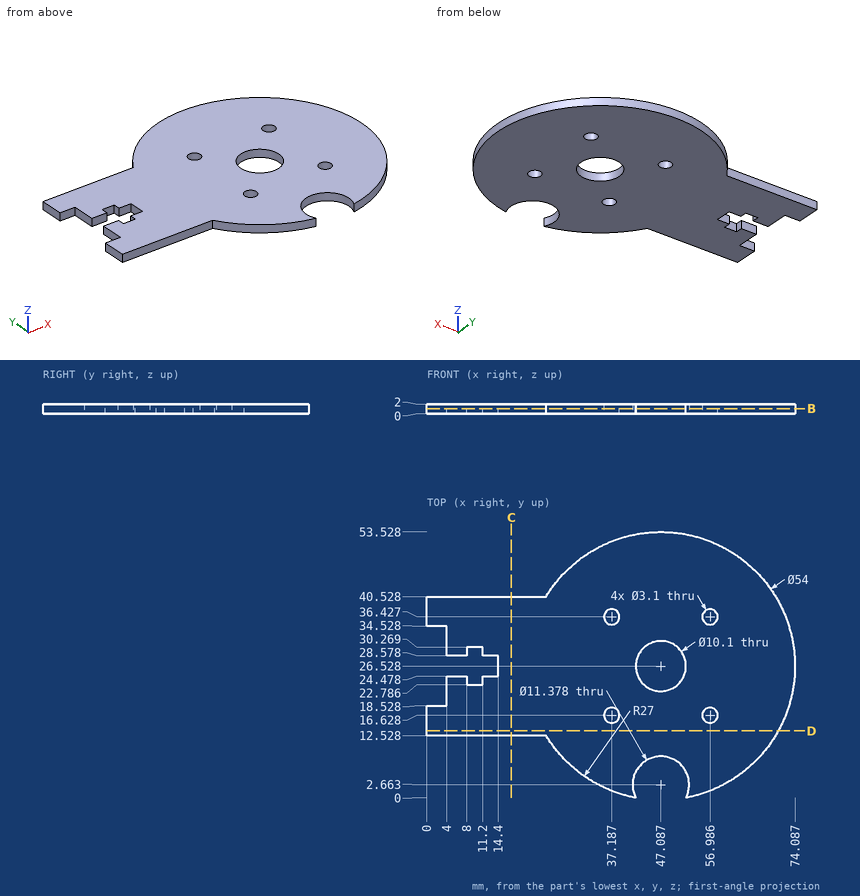
Print and shaded views of the part. All mm, measured from the part's lowest x, y and z. Round coordinates to 2 decimals unless told otherwise and drop trailing zeros. Write each loop counter-clockwise with the first axis right and the second up, starting at its lowest first coordinate (ties: lowest second). Pieces come first, ordered by that corner, then holes. Notation, with made-up numbers: M 84.25,70 L 141.25,70 A16 ccw 141.25,92 Z; hole C 52,87 d2. An arc over 180 degrees is marked long. Use a Markdown table: item, result. Add a question column.
1. Slice it at C-C on x = 17. Give the cut face in (y, z).
2. Drill centre lines: probe 1 along X at (y, z) = (37, 1) (1 decimal); probe 2 along Y at (x, z) = (5.5, 0.7); probe 3 along X at (y, z) = (37.5, 1.25) (1 decimal). Where is each one in solid material? Low to high.
3. Flat gauge pins, fed straight in: P1, Ø11.5, axis at x = 47.09, y = 26.53, coming from the -Z side; P2, Ø1, axis at y = 32.5, z = 1, coming from the -X side; P3, Ø1.9, axis at x = 56.99, y = 36.43, coming from the +Z side; P4, Ø1, axis at y = 26, z = 1, coming from the -X side. Where does each tip first touch, or does it go through?
4. Slice it at D-D on y = 13.5. Give the cut face in (x, z) (1 decimal).
5. Slice it at B-B on z = 1.05. Give the number of separate pieces and of enclosed holes in the cut face, then the cut area to 3 significant figures.
Reply:
| question | item | result |
|---|---|---|
| 1 | outline | M 12.53,0 L 40.53,0 L 40.53,2 L 12.53,2 Z |
| 2 | probe 1 | x = 0 to 35.7, 38.6 to 55.5, 58.4 to 72 |
| 2 | probe 2 | y = 12.53 to 24.48, 28.58 to 40.53 |
| 2 | probe 3 | x = 0 to 36.1, 38.3 to 55.9, 58.1 to 71.8 |
| 3 | P1 | stops at z = 0 |
| 3 | P2 | stops at x = 4 |
| 3 | P3 | passes through |
| 3 | P4 | stops at x = 14.4 |
| 4 | outline | M 0,0 L 70.7,0 L 70.7,2 L 0,2 Z |
| 5 | separate pieces | 1 |
| 5 | enclosed holes | 5 |
| 5 | area | 2,580 mm^2 |
